For this review, take the finished solid that the model builds, in its own axes (mm). Coordinates: 2 decimals unless noted, no trailing zeros. Loops run counter-clockwise (first coordinate to the right, second up) from the corner with the lowest first, then second, coordinate; pieces in that order, holes last. Notation, with made-up numbers: M -26.75,87 L -8.75,87 A21 ccw -8.75,115 Z; hole C 32.5,-5.5 d7. An arc over 180 degrees is marked long. Put each result on its own line as item: value.
```python
from build123d import *

# Parameters (mm, degrees)
SKETCH_1_R          = 2.45875
EXTRUDE_555_DEPTH   = 6.7
SKETCH_2_OUTSIDE_W  = 52.598
SKETCH_2_OUTSIDE_H  = 54.078
SKETCH_2_OUTSIDE_R  = 5
CUT_EXTRUDE_1_DEPTH = 10.915132059
CUT_EXTRUDE_1_DRAFT = -60
CHAMFER_1_SIZE      = 0.129464286
SKETCH_9_OUTSIDE_W  = 36.616
SKETCH_9_OUTSIDE_H  = 38.096
SKETCH_9_OUTSIDE_R  = 4.5
CUT_EXTRUDE_7_DEPTH = 10.915132059
CUT_EXTRUDE_7_DRAFT = -45


with BuildPart() as part:
    # 草图1 → Extrude 555 (new body)
    with BuildSketch(Plane.XY):
        Polygon((0, 5.525), (-4.784790356, 2.7625), (-4.784790356, -2.7625), (0, -5.525), (4.784790356, -2.7625), (4.784790356, 2.7625), align=None)
        Circle(SKETCH_1_R, mode=Mode.SUBTRACT)
    extrude(amount=EXTRUDE_555_DEPTH)


with BuildPart() as cut_extrude_1_tool:
    # 草图2 outside → 切除-拉伸1 (with draft: the straight prism first)
    with BuildSketch(Plane(origin=(0, 0, 0), x_dir=(-1, 0, 0), z_dir=(0, 0, -1))):
        Rectangle(SKETCH_2_OUTSIDE_W, SKETCH_2_OUTSIDE_H)
        Circle(SKETCH_2_OUTSIDE_R, mode=Mode.SUBTRACT)
    extrude(amount=-CUT_EXTRUDE_1_DEPTH)
    # 切除-拉伸1: the draft: its side faces are tilted about the plane it starts from
    cut_extrude_1_sides = [cut_extrude_1_tool.faces().sort_by_distance(p)[0] for p in [
        (0, -27.039, 5.45756603),
        (-26.299, 0, 5.45756603),
        (0, 27.039, 5.45756603),
        (26.299, 0, 5.45756603),
        (5, 0, 5.45756603),
    ]]
    draft(cut_extrude_1_sides, Plane(origin=(0, 0, 0), x_dir=(-1, 0, 0), z_dir=(0, 0, -1)), CUT_EXTRUDE_1_DRAFT)


with BuildPart() as part_1:
    add(part.part)

    # 切除-拉伸1: cut by cut_extrude_1_tool
    add(cut_extrude_1_tool.part, mode=Mode.SUBTRACT)

    # 倒角1
    chamfer_1_edges = [part_1.edges().sort_by_distance(p)[0] for p in [
        (-2.45875, 0, 0),
    ]]
    chamfer(chamfer_1_edges, length=CHAMFER_1_SIZE)


with BuildPart() as cut_extrude_7_tool:
    # 草图9 outside → 切除-拉伸7 (with draft: the straight prism first)
    with BuildSketch(Plane.XY.offset(6.7)):
        Rectangle(SKETCH_9_OUTSIDE_W, SKETCH_9_OUTSIDE_H)
        Circle(SKETCH_9_OUTSIDE_R, mode=Mode.SUBTRACT)
    extrude(amount=-CUT_EXTRUDE_7_DEPTH)
    # 切除-拉伸7: the draft: its side faces are tilted about the plane it starts from
    cut_extrude_7_sides = [cut_extrude_7_tool.faces().sort_by_distance(p)[0] for p in [
        (0, -19.048, 1.24243397),
        (18.308, 0, 1.24243397),
        (0, 19.048, 1.24243397),
        (-18.308, 0, 1.24243397),
        (-4.5, 0, 1.24243397),
    ]]
    draft(cut_extrude_7_sides, Plane.XY.offset(6.7), CUT_EXTRUDE_7_DRAFT)


with BuildPart() as part_2:
    add(part_1.part)

    # 切除-拉伸7: cut by cut_extrude_7_tool
    add(cut_extrude_7_tool.part, mode=Mode.SUBTRACT)


solid = part_2.part
```
(1) Wall thickness on line 1 along Y through (x, z) = (-1.5, 3.75); line 2 along Y through (x, z) = (-2, 0.5); line 3 along X through (y, z) = (2, 3.25): over which ranges is each line inside the solid? List them lowest first. Write a range as [from, to].
Determined:
line 1: y = [-4.66, -1.95], [1.95, 4.66]
line 2: y = [-4.37, -1.43], [1.43, 4.37]
line 3: x = [-4.78, -1.43], [1.43, 4.78]
(2) Add section A-A (y = 0). Write out the cut boundary in (x, z).
Determined:
outline: M -4.78,0 L -2.59,0 L -2.46,0.13 L -2.46,6.7 L -4.5,6.7 L -4.78,6.42 Z; M 2.46,0.13 L 2.59,0 L 4.78,0 L 4.78,6.42 L 4.5,6.7 L 2.46,6.7 Z
(3) For pin 1 (1 mm diameter, centred on x = 1, z = 5.5, fed in from -Y), flat-tipped, find the tip position at first contact; note if it passes through.
Determined:
pin 1: stops at y = -5.24
(4) Add section B-B (z = 3.25). Write out the cut boundary in (x, y) (1 decimal).
Determined:
outline: M -4.8,-2.8 L 0,-5.5 L 4.8,-2.8 L 4.8,2.8 L 0,5.5 L -4.8,2.8 Z; hole C 0,0 d4.9
(5) Draft analysis for pull direction X (two halves, no side actions). For faces 1 (the cylindrical face through (2.345, 0.739, 3.369)), 2 (the flat face through (-2.43, -4.12, 3.16)), 3 (the flat face through (4.785, 0, 3)), 4 (the flat face through (-2, -2, 0)), state which applies: +X half, -X half, draft (parallel to the pull), parting line (faces both ways), or undercut.
Determined:
face 1: undercut
face 2: -X half
face 3: +X half
face 4: draft
